Check sheet for the modelled part. Datum: model origin and axes. Units: mm. Coordinates: 2 decimals unless noted, no trailing zeros. Order: outer loops, then holes, each group sorted by start corner. A loop starts at its lowest first (then second) coordinate and runs counter-clockwise, first axis right, second up.
from build123d import *

# Parameters (mm, degrees)
SKETCH_1_R      = 1.503661285
SKETCH_1_R_2    = 1.504036587
EXTRUDE_1_DEPTH = 3


with BuildPart() as part:
    # 草图1 → 凸台-拉伸1 (new body)
    with BuildSketch(Plane.XY):
        with BuildLine():
            Line((0, 0), (15.002289805, 0))
            ThreePointArc((15.002289805, 0), (16.770627342, -4.269144464), (12.501482877, -2.500806927))
            Line((12.501482877, -2.500806927), (-12.497361882, -2.500806927))
            ThreePointArc((-12.497361882, -2.500806927), (-16.766506346, -4.269144464), (-14.998168809, 0))
            Line((-14.998168809, 0), (0, 0))
        make_face()
        with Locations((-14.998168809, -2.500806927)):
            Circle(SKETCH_1_R, mode=Mode.SUBTRACT)
        with Locations((15.002289805, -2.500806927)):
            Circle(SKETCH_1_R_2, mode=Mode.SUBTRACT)
    extrude(amount=EXTRUDE_1_DEPTH)


solid = part.part
(1) Cross-section at D-D (x = 15.5). Enter the section's corners in (y, z).
Filled in:
outline: (-4.95, 0) - (-3.92, 0) - (-3.92, 3) - (-4.95, 3) - close; (-1.08, 0) - (-0.05, 0) - (-0.05, 3) - (-1.08, 3) - close
(2) Cross-section at B-B (y = -1.75). Enter the section's corners in (x, z).
Filled in:
outline: (-17.38, 0) - (-16.3, 0) - (-16.3, 3) - (-17.38, 3) - close; (-13.7, 0) - (13.7, 0) - (13.7, 3) - (-13.7, 3) - close; (16.31, 0) - (17.39, 0) - (17.39, 3) - (16.31, 3) - close
(3) Cross-section at A-A (z = 0.5). Enter the section's corners in (x, y), and give its area (3 significant figures).
Filled in:
outline: (-15, 0) arc R2.5 ccw (long way) to (-12.5, -2.5) - (12.5, -2.5) arc R2.5 ccw (long way) to (15, 0) - close; hole circle Ø3.01 at (-15, -2.5); hole circle Ø3.01 at (15, -2.5)
area: 90.3 mm2
(4) Thickness scan on probe 1 along X at (y, z) = (-3.7, 2.85); probe 2 along X at (y, z) = (-1.45, 1.45); probe 3 along X at (y, z) = (-3.8, 0.7). Record the ranges inside material, lowest first.
Filled in:
probe 1: x = -17.19 to -15.91, -14.09 to -12.8, 12.81 to 14.09, 15.91 to 17.2
probe 2: x = -17.27 to -16.07, -13.92 to 13.93, 16.08 to 17.27
probe 3: x = -17.14 to -15.76, -14.24 to -12.86, 12.87 to 14.24, 15.76 to 17.14
(5) Go/stop test with a flat-tipped pin: P1, Ø1.5, axis at x = 3, z = 1.5, coming from the -Y side. Record where the tip stops, or that it passes through.
Filled in:
P1: stops at y = -2.5
(6) Cross-section at C-C (y = -3.5). Enter the section's corners in (x, z).
Filled in:
outline: (-17.29, 0) - (-16.12, 0) - (-16.12, 3) - (-17.29, 3) - close; (-13.87, 0) - (-12.71, 0) - (-12.71, 3) - (-13.87, 3) - close; (12.71, 0) - (13.88, 0) - (13.88, 3) - (12.71, 3) - close; (16.13, 0) - (17.29, 0) - (17.29, 3) - (16.13, 3) - close
(7) Release check for a two-part mould opening along X. For faces 1 (the cylindrical face through (-13.61, -3.08, 1.48)), 2 (the flat face through (0, -2.501, 1)), 3 (the flat face through (0, 0, 1)) record: +X half, -X half, draft (parallel to the pull), parting line (faces both ways), or undercut.
Filled in:
face 1: undercut
face 2: undercut
face 3: draft
